Check sheet for the modelled part. Datum: model origin and axes. Units: mm. Face numbers are marked on the shaded views. A direction names the side the tool comes from. Round coordinates to 2 decimals unless told otherwise and drop trailing zeros. Loops run counter-clockwise (first coordinate to the right, second up) from the corner with the lowest first, then second, coordinate; pieces in that order, holes last. Notation, with made-up numbers: (87.25, 64.5) -> (114.25, 64.5) arc R8 ccw to (114.25, 78.5) -> close; hole circle Ø10 at (63.25, -19). An arc over 180 degrees is marked (long way). Use one line per item in the form item = value. Start each with the question number.
(1) Sectioned sample at C-C (z = 14.5). Record the cut outline in (x, y), and give its area (3 significant figures).
(2) Material ranges on probe 1 along Y at (x, z) = (10, 2); probe 2 along Y at (x, z) = (1, 12); probe 3 along Y at (x, z) = (7, 9), recorded low to high. Write a range as [from, to].
(3) Sectioned sample at A-A (x = 10). Record the cut outline in (y, z).
(4) Sectioned sample at B-B (x = 0). Record the cut outline in (y, z).
(5) Sectioned sample at D-D (y = -13). Record the cut outline in (x, z).
(6) Set-up check for the marked faces 1 and 2: record each of +Z, -Z, +X, -X, +Y, -Y from which the full face is reachable in a straight line by a thin tool's end or side.
(7) Go/stop test with flat-tipped pins: pin 1 (1 mm diameter, centred on x = -13.5, z = -6.5, fed in from -Y); pin 2 (8 mm diameter, centred on y = -11, z = -5.5, fed in from +X); pin 3 (3 mm diameter, centred on x = 1.5, y = -11.5, fed in from -Z); pin 4 (3 mm diameter, centred on x = 14.5, z = -13.5, fed in from -Y). Record where each tip stops, or that it passes through.
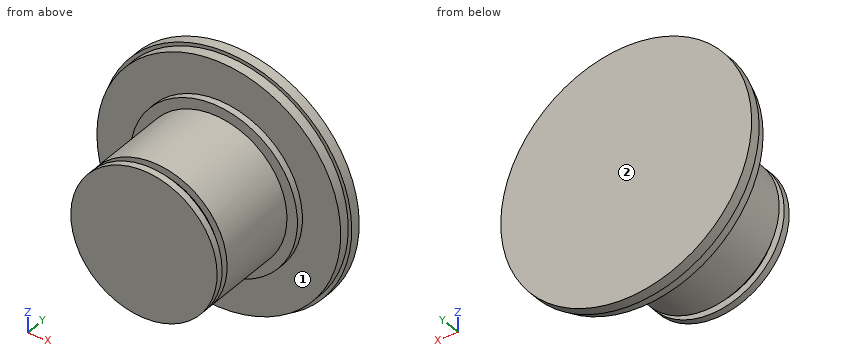
from build123d import *

# Parameters (mm, degrees)
SKETCH1_R           = 18
BOSS_EXTRUDE1_DEPTH = 1.5
SKETCH2_R           = 17.5
BOSS_EXTRUDE2_DEPTH = 1.5
SKETCH3_R           = 12
BOSS_EXTRUDE3_DEPTH = 1
SKETCH4_R           = 10.5
BOSS_EXTRUDE4_DEPTH = 12
SKETCH5_R           = 9.5
BOSS_EXTRUDE5_DEPTH = 1
SKETCH6_R           = 10.5
BOSS_EXTRUDE6_DEPTH = 1


with BuildPart() as part:
    # Sketch1 → Boss-Extrude1 (new body)
    with BuildSketch(Plane(origin=(0, 0, 0), x_dir=(1, 0, 0), z_dir=(0, 1, 0))):
        with Locations(Location((0, 0, 0), (0, 0, 270))):
            Circle(SKETCH1_R)
    extrude(amount=BOSS_EXTRUDE1_DEPTH)

    # Sketch2 → Boss-Extrude2 (add)
    with BuildSketch(Plane.XZ):
        with Locations(Location((0, 0, 0), (0, 0, 270))):
            Circle(SKETCH2_R)
    extrude(amount=BOSS_EXTRUDE2_DEPTH)

    # Sketch3 → Boss-Extrude3 (add)
    with BuildSketch(Plane.XZ.offset(1.5)):
        with Locations(Location((0, 0, 0), (0, 0, 270))):
            Circle(SKETCH3_R)
    extrude(amount=BOSS_EXTRUDE3_DEPTH)

    # Sketch4 → Boss-Extrude4 (add)
    with BuildSketch(Plane.XZ.offset(2.5)):
        with Locations(Location((0, 0, 0), (0, 0, 270))):
            Circle(SKETCH4_R)
    extrude(amount=BOSS_EXTRUDE4_DEPTH)

    # Sketch5 → Boss-Extrude5 (add)
    with BuildSketch(Plane.XZ.offset(14.5)):
        with Locations(Location((0, 0, 0), (0, 0, 270))):
            Circle(SKETCH5_R)
    extrude(amount=BOSS_EXTRUDE5_DEPTH)

    # Sketch6 → Boss-Extrude6 (add)
    with BuildSketch(Plane.XZ.offset(15.5)):
        with Locations(Location((0, 0, 0), (0, 0, 270))):
            Circle(SKETCH6_R)
    extrude(amount=BOSS_EXTRUDE6_DEPTH)


solid = part.part
Checks:
q1.outline = (-10.67, 0) -> (-9.8, 0) -> (-9.8, -1.5) -> (9.8, -1.5) -> (9.8, 0) -> (10.67, 0) -> (10.67, 1.5) -> (-10.67, 1.5) -> close
q1.area = 61.4 mm2
q2.probe_1 = [-16.5, -15.5], [-14.5, 1.5]
q2.probe_2 = [-1.5, 1.5]
q2.probe_3 = [-2.5, 1.5]
q3.outline = (-16.5, -3.2) -> (-15.5, -3.2) -> (-15.5, 3.2) -> (-16.5, 3.2) -> close; (-14.5, -3.2) -> (-2.5, -3.2) -> (-2.5, -6.63) -> (-1.5, -6.63) -> (-1.5, -14.36) -> (0, -14.36) -> (0, -14.97) -> (1.5, -14.97) -> (1.5, 14.97) -> (0, 14.97) -> (0, 14.36) -> (-1.5, 14.36) -> (-1.5, 6.63) -> (-2.5, 6.63) -> (-2.5, 3.2) -> (-14.5, 3.2) -> close
q4.outline = (-16.5, -10.5) -> (-15.5, -10.5) -> (-15.5, -9.5) -> (-14.5, -9.5) -> (-14.5, -10.5) -> (-2.5, -10.5) -> (-2.5, -12) -> (-1.5, -12) -> (-1.5, -17.5) -> (0, -17.5) -> (0, -18) -> (1.5, -18) -> (1.5, 18) -> (0, 18) -> (0, 17.5) -> (-1.5, 17.5) -> (-1.5, 12) -> (-2.5, 12) -> (-2.5, 10.5) -> (-14.5, 10.5) -> (-14.5, 9.5) -> (-15.5, 9.5) -> (-15.5, 10.5) -> (-16.5, 10.5) -> close
q5.outline = circle Ø21 at (0, 0)
q6.face_1 = -Y
q6.face_2 = +Z, -Z, +X, -X, +Y
q7.pin_1 = -1.5
q7.pin_2 = 10.39
q7.pin_3 = -10.5
q7.pin_4 = through
